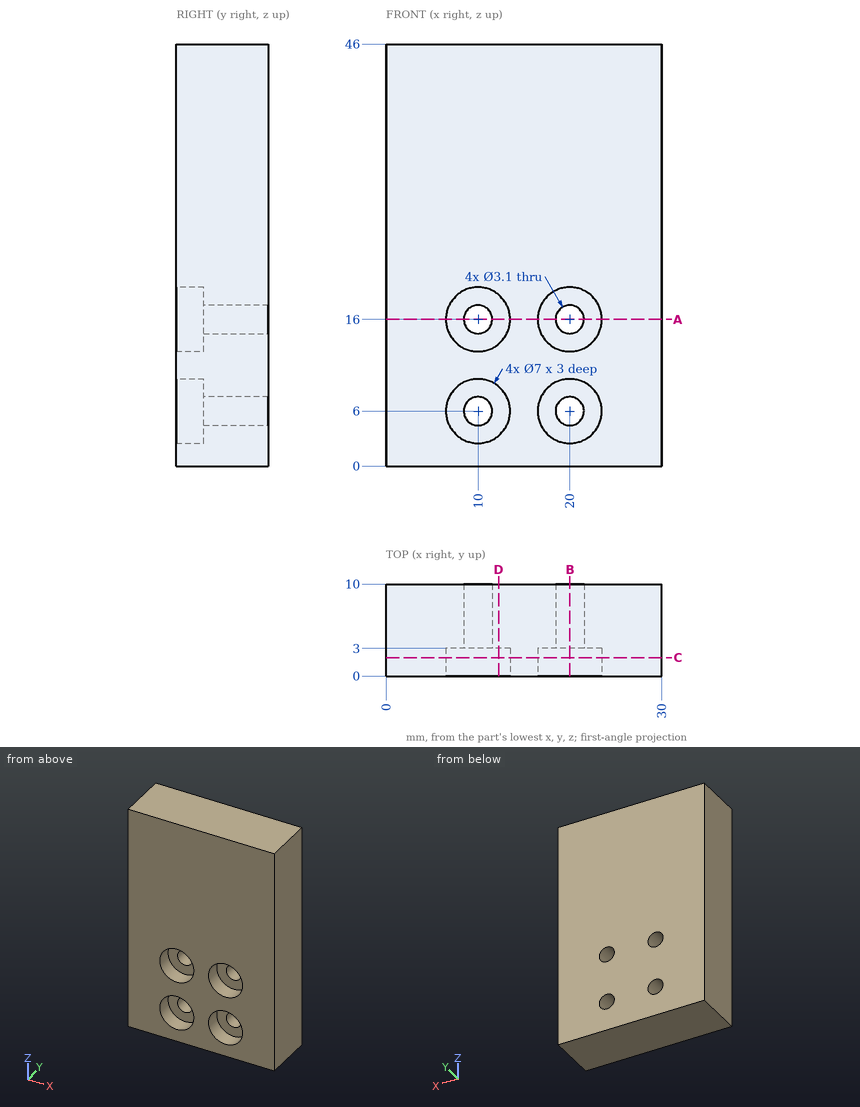
Drawing for the job (mm, zero at the part's lowest x, y, z). Give positions to 0.01 mm unless a question says otherwise; leave off trailing zeros. Write each loop counter-clockwise with the first axis right and the second up, starting at its lowest first coordinate (ties: lowest second). Pieces come first, ordered by that corner, then holes. Notation, with made-up numbers: (5, 11.25) -> (18, 11.25) arc R27 ccw to (18, 48.25) -> close; hole circle Ø3 at (54, -4.5). An arc over 180 degrees is marked (long way). Put each result on its own line as item: value. Start each with the question number.
Item 1: Cut at A-A (z = 16). List the corners of the cut face in (x, y).
Item 2: Wall check: L1, parallel to X at y = 1.75, z = 6; L2, parallel to X at y = 4.5, z = 6; L3, parallel to Z at x = 17.25, y = 1.75. Give the ranges that are in metal, low to high. Write a range as [from, to].
Item 3: Cut at D-D (x = 12.25). List the corners of the cut face in (y, z), then the cut area to 3 significant figures.
Item 4: Pin check, flat tips, straight feed: pin 1 Ø3 at (x, z) = (10, 6) entering from -Y; pin 2 Ø2 at (x, z) = (18.5, 5.5) entering from -Y. Stop position of each tip, or through.
Item 5: Cut at B-B (x = 20). List the corners of the cut face in (y, z), then the cut area to 3 significant figures.
Item 6: Cut at C-C (y = 2). List the corners of the cut face in (x, z).
Answer list:
1. outline: (0, 0) -> (6.5, 0) -> (6.5, 3) -> (8.45, 3) -> (8.45, 10) -> (0, 10) -> close; (11.55, 3) -> (13.5, 3) -> (13.5, 0) -> (16.5, 0) -> (16.5, 3) -> (18.45, 3) -> (18.45, 10) -> (11.55, 10) -> close; (21.55, 3) -> (23.5, 3) -> (23.5, 0) -> (30, 0) -> (30, 10) -> (21.55, 10) -> close
2. L1: x = [0, 6.5], [13.5, 16.5], [23.5, 30]
2. L2: x = [0, 8.45], [11.55, 18.45], [21.55, 30]
2. L3: z = [0, 3.83], [8.17, 13.83], [18.17, 46]
3. outline: (0, 0) -> (10, 0) -> (10, 46) -> (0, 46) -> (0, 18.68) -> (3, 18.68) -> (3, 13.32) -> (0, 13.32) -> (0, 8.68) -> (3, 8.68) -> (3, 3.32) -> (0, 3.32) -> close
3. area: 428 mm2
4. pin 1: passes through
4. pin 2: stops at y = 3
5. outline: (0, 0) -> (10, 0) -> (10, 4.45) -> (3, 4.45) -> (3, 2.5) -> (0, 2.5) -> close; (0, 9.5) -> (3, 9.5) -> (3, 7.55) -> (10, 7.55) -> (10, 14.45) -> (3, 14.45) -> (3, 12.5) -> (0, 12.5) -> close; (0, 19.5) -> (3, 19.5) -> (3, 17.55) -> (10, 17.55) -> (10, 46) -> (0, 46) -> close
5. area: 375 mm2
6. outline: (0, 0) -> (30, 0) -> (30, 46) -> (0, 46) -> close; hole circle Ø7 at (10, 6); hole circle Ø7 at (10, 16); hole circle Ø7 at (20, 6); hole circle Ø7 at (20, 16)
